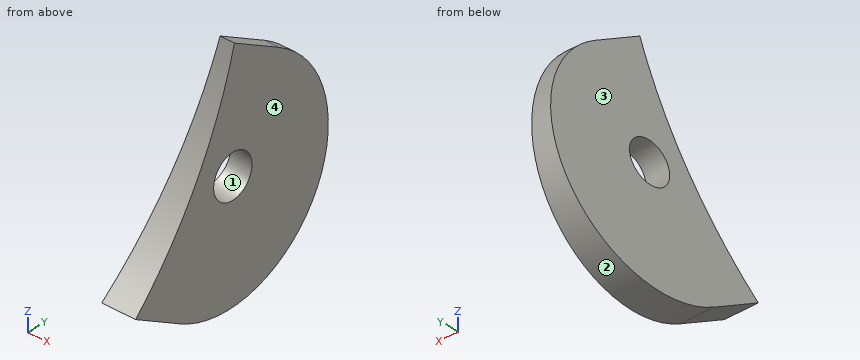
```python
from build123d import *

# Parameters (mm, degrees)
PAD040_DEPTH         = 42
SKETCH121_W          = 51.449978
SKETCH121_H          = 41.216857
POCKET061_DEPTH      = 2.357074
POCKET061_DEPTH_BACK = 0.001
SKETCH122_R          = 1.5
POCKET062_DEPTH      = 9.321248
POCKET062_DEPTH_BACK = 0.001


with BuildPart() as part:
    # Sketch120 (on DatumPlane) → Pad040 (new body)
    with BuildSketch(Plane(origin=(6, 0, 0), x_dir=(1, 0, 0), z_dir=(0, -0.866025, 0.5))):
        Polygon((-6, 7.75), (-6, -7.75), (-8.356074, -7.75), (-7, 7.75), align=None)
    extrude(amount=-PAD040_DEPTH)

    # Sketch121 → Pocket061 (cut, two sides)
    with BuildSketch(Plane.YZ) as pocket061_sk:
        with Locations((16.010519, -12.541656)):
            Rectangle(SKETCH121_W, SKETCH121_H)
        with BuildLine():
            ThreePointArc((21.223867, -21.202535), (25.980762, -15), (28.973867, -7.779141))
            Line((28.973867, -7.779141), (32.453838, -9.788303))
            ThreePointArc((24.703838, -23.211697), (35.290535, -20.375), (32.453838, -9.788303))
            Line((21.223867, -21.202535), (24.703838, -23.211697))
        make_face(mode=Mode.SUBTRACT)
    extrude(amount=-POCKET061_DEPTH, mode=Mode.SUBTRACT)
    extrude(pocket061_sk.sketch, amount=POCKET061_DEPTH_BACK, mode=Mode.SUBTRACT)

    # Sketch122 (on DatumPlane) → Pocket062 (cut, two sides)
    with BuildSketch(Plane(origin=(6, 0, 0), x_dir=(0.087156, 0.498097, 0.86273), z_dir=(0.996195, -0.043578, -0.075479))) as pocket062_sk:
        with Locations((0, -33)):
            Circle(SKETCH122_R)
    extrude(amount=-POCKET062_DEPTH, mode=Mode.SUBTRACT)
    extrude(pocket062_sk.sketch, amount=POCKET062_DEPTH_BACK, mode=Mode.SUBTRACT)


with BuildPart() as part_1:
    # Body022023 placement: moved
    add(part.part.moved(Location((123, 0, 835))))


solid = part_1.part
```
The listing builds one solid part. Answer for the finished solid, in the listing's coordinates (mm). Face numbers are marked on the shaded views. Coordinates: 2 decimals unless noted, no trailing zeros. Loops run counter-clockwise (first coordinate to the right, second up) from the corner with the lowest first, then second, coordinate; pieces in that order, holes last. Notation, with made-up numbers: (25.5, 69) -> (66.5, 69) arc R20 ccw to (66.5, 92) -> close; hole circle Ø4 at (-28, -18). An arc over 180 degrees is marked (long way). Use one line per item in the form item = value. Start each with the question number.
Item 1: The mould has two halves that part along Z. Classify the marked faces 1, 2, 3 and 4: released by +Z, released by -Z, zero draft, split by the parting line, or undercut.
Item 2: The part is cut by section B-B on x = 120.95. Determine the outline of the cut face in (y, z).
Item 3: Consider L1, parallel to X at y = 26.75, z = 811.5; L2, parallel to Y at x = 121.35, z = 814; L3, parallel to Z at x = 122.8, y = 26.5. Determine where each line is inside the solid, lowest interval first. Write a range as [from, to].
Item 4: The part is cut by section A-A on y = 24. Determine the outline of the cut face in (x, z).
Answer key:
q1.face_1 = undercut
q1.face_2 = split by the parting line
q1.face_3 = released by +Z
q1.face_4 = zero draft
q2.outline = (21.22, 813.8) -> (24.7, 811.79) arc R7.75 ccw to (32.06, 811.58) -> (23.59, 816.47) arc R30 cw to start
q3.L1 = [120.71, 123]
q3.L2 = [21.42, 34.89]
q3.L3 = [811.03, 820.94]
q4.outline = (120.64, 812.19) -> (123, 812.19) -> (123, 817) -> (121.01, 817) -> close
